from build123d import *

# Parameters (mm, degrees)
SKETCH1_W          = 432
SKETCH1_H          = 255
BASE_FLANGE1_DEPTH = 4
SKETCH4_R          = 1.75
SKETCH4_W          = 4
SKETCH4_H          = 40
SKETCH4_W_2        = 6.3
CUT_EXTRUDE1_DEPTH = 251.855037821
CUT_EXTRUDE2_DEPTH = 251.855037821
SKETCH6_R          = 1.75
CUT_EXTRUDE3_DEPTH = 251.855037821
CUT_EXTRUDE4_REACH = 252.855
SKETCH7_R          = 2.25
SKETCH8_R          = 3.25
CUT_EXTRUDE5_DEPTH = 251.855037821
CUT_EXTRUDE6_DEPTH = 251.855037821
SKETCH10_W         = 4
SKETCH10_H         = 100
CUT_EXTRUDE7_DEPTH = 251.855037821
CUT_EXTRUDE8_DEPTH = 251.855037821
SKETCH13_W         = 4
SKETCH13_H         = 20.5
TAB1_DEPTH         = 4
CUT_EXTRUDE9_REACH = 252.855


# Sheet-metal steps are written as plain solids
with BuildPart() as part:
    # Sketch1 → Base-Flange1 (new body)
    with BuildSketch(Plane.XY):
        Rectangle(SKETCH1_W, SKETCH1_H)
    extrude(amount=-BASE_FLANGE1_DEPTH)

    # Sketch4 → Cut-Extrude1 (cut, through all)
    with BuildSketch(Plane.XY):
        with Locations((-78, 82.5)):
            Circle(SKETCH4_R)
        with Locations(Location((214, -17.5, 0), (0, 0, 180))):
            Circle(SKETCH4_R)
        with Locations(Location((214, 82.5, 0), (0, 0, 180))):
            Circle(SKETCH4_R)
        with Locations((-78, -17.5)):
            Circle(SKETCH4_R)
        with Locations((-169, -17.5)):
            Circle(SKETCH4_R)
        with Locations((-169, 82.5)):
            Circle(SKETCH4_R)
        with Locations((-214, 82.5)):
            Circle(SKETCH4_R)
        with Locations((-214, -17.5)):
            Circle(SKETCH4_R)
        with Locations(Location((169, 82.5, 0), (0, 0, 180))):
            Circle(SKETCH4_R)
        with Locations(Location((169, -17.5, 0), (0, 0, 180))):
            Circle(SKETCH4_R)
        with Locations(Location((78, -17.5, 0), (0, 0, 180))):
            Circle(SKETCH4_R)
        with Locations(Location((78, 82.5, 0), (0, 0, 180))):
            Circle(SKETCH4_R)
        with Locations((-214, 32.5)):
            Rectangle(SKETCH4_W, SKETCH4_H)
        with Locations((-169, 32.5)):
            Rectangle(SKETCH4_W_2, SKETCH4_H)
        with Locations((-78, 32.5)):
            Rectangle(SKETCH4_W_2, SKETCH4_H)
        with Locations((78, 32.5)):
            Rectangle(SKETCH4_W_2, SKETCH4_H)
        with Locations((169, 32.5)):
            Rectangle(SKETCH4_W_2, SKETCH4_H)
        with Locations((214, 32.5)):
            Rectangle(SKETCH4_W, SKETCH4_H)
    extrude(amount=-CUT_EXTRUDE1_DEPTH, mode=Mode.SUBTRACT)

    # Sketch5 → Cut-Extrude2 (cut, through all)
    with BuildSketch(Plane.XY):
        with BuildLine():
            Line((-214, 80.75), (-216, 80.75))
            ThreePointArc((-216, 80.75), (-217.75, 82.5), (-216, 84.25))
            Line((-216, 84.25), (-214, 84.25))
            ThreePointArc((-214, 84.25), (-212.25, 82.5), (-214, 80.75))
        make_face()
        with BuildLine():
            Line((-214, -19.25), (-216, -19.25))
            ThreePointArc((-216, -19.25), (-217.75, -17.5), (-216, -15.75))
            Line((-216, -15.75), (-214, -15.75))
            ThreePointArc((-214, -15.75), (-212.25, -17.5), (-214, -19.25))
        make_face()
        with BuildLine():
            Line((214, 80.75), (216, 80.75))
            ThreePointArc((216, 80.75), (217.75, 82.5), (216, 84.25))
            Line((216, 84.25), (214, 84.25))
            ThreePointArc((214, 84.25), (212.25, 82.5), (214, 80.75))
        make_face()
        with BuildLine():
            Line((214, -19.25), (216, -19.25))
            ThreePointArc((216, -19.25), (217.75, -17.5), (216, -15.75))
            Line((216, -15.75), (214, -15.75))
            ThreePointArc((214, -15.75), (212.25, -17.5), (214, -19.25))
        make_face()
    extrude(amount=-CUT_EXTRUDE2_DEPTH, mode=Mode.SUBTRACT)

    # Sketch6 → Cut-Extrude3 (cut, through all)
    with BuildSketch(Plane.XY):
        with Locations((-90, -54.5)):
            Circle(SKETCH6_R)
        with Locations((90, -54.5)):
            Circle(SKETCH6_R)
    extrude(amount=-CUT_EXTRUDE3_DEPTH, mode=Mode.SUBTRACT)

    # Sketch7 → Cut-Extrude4 (cut, up to next)
    with BuildSketch(Plane.XY, mode=Mode.PRIVATE) as cut_extrude4_sk1:
        with Locations((205.5, 115.5)):
            Circle(SKETCH7_R)
    cut_extrude4_tool1 = extrude(cut_extrude4_sk1.sketch, amount=-CUT_EXTRUDE4_REACH, mode=Mode.PRIVATE) & part.part
    # Sketch7 → Cut-Extrude4 (cut, up to next)
    with BuildSketch(Plane.XY, mode=Mode.PRIVATE) as cut_extrude4_sk2:
        with Locations((205.5, 99.5)):
            Circle(SKETCH7_R)
    cut_extrude4_tool2 = extrude(cut_extrude4_sk2.sketch, amount=-CUT_EXTRUDE4_REACH, mode=Mode.PRIVATE) & part.part
    # Sketch7 → Cut-Extrude4 (cut, up to next)
    with BuildSketch(Plane.XY, mode=Mode.PRIVATE) as cut_extrude4_sk3:
        with Locations((-205.5, 99.5)):
            Circle(SKETCH7_R)
    cut_extrude4_tool3 = extrude(cut_extrude4_sk3.sketch, amount=-CUT_EXTRUDE4_REACH, mode=Mode.PRIVATE) & part.part
    # Sketch7 → Cut-Extrude4 (cut, up to next)
    with BuildSketch(Plane.XY, mode=Mode.PRIVATE) as cut_extrude4_sk4:
        with Locations((-205.5, 115.5)):
            Circle(SKETCH7_R)
    cut_extrude4_tool4 = extrude(cut_extrude4_sk4.sketch, amount=-CUT_EXTRUDE4_REACH, mode=Mode.PRIVATE) & part.part
    add(cut_extrude4_tool1.solids().sort_by_distance((205.5, 115.5, 0))[0], mode=Mode.SUBTRACT)
    add(cut_extrude4_tool2.solids().sort_by_distance((205.5, 99.5, 0))[0], mode=Mode.SUBTRACT)
    add(cut_extrude4_tool3.solids().sort_by_distance((-205.5, 99.5, 0))[0], mode=Mode.SUBTRACT)
    add(cut_extrude4_tool4.solids().sort_by_distance((-205.5, 115.5, 0))[0], mode=Mode.SUBTRACT)

    # Sketch8 → Cut-Extrude5 (cut, through all)
    with BuildSketch(Plane.XY):
        with Locations((-143.5, -67.5)):
            Circle(SKETCH8_R)
        with Locations((-103.5, -67.5)):
            Circle(SKETCH8_R)
        with Locations((-20, -67.5)):
            Circle(SKETCH8_R)
        with Locations((20, -67.5)):
            Circle(SKETCH8_R)
        with Locations((103.5, -67.5)):
            Circle(SKETCH8_R)
        with Locations((143.5, -67.5)):
            Circle(SKETCH8_R)
    extrude(amount=-CUT_EXTRUDE5_DEPTH, mode=Mode.SUBTRACT)

    # Sketch9 → Cut-Extrude6 (cut, through all)
    with BuildSketch(Plane.XY):
        with BuildLine():
            Line((-143.5, -77.5), (-103.5, -77.5))
            ThreePointArc((-103.5, -77.5), (-93.5, -87.5), (-103.5, -97.5))
            Line((-103.5, -97.5), (-143.5, -97.5))
            ThreePointArc((-143.5, -97.5), (-153.5, -87.5), (-143.5, -77.5))
        make_face()
        with BuildLine():
            Line((-20, -77.5), (20, -77.5))
            ThreePointArc((20, -77.5), (30, -87.5), (20, -97.5))
            Line((20, -97.5), (-20, -97.5))
            ThreePointArc((-20, -97.5), (-30, -87.5), (-20, -77.5))
        make_face()
        with BuildLine():
            Line((143.5, -77.5), (103.5, -77.5))
            ThreePointArc((103.5, -77.5), (93.5, -87.5), (103.5, -97.5))
            Line((103.5, -97.5), (143.5, -97.5))
            ThreePointArc((143.5, -97.5), (153.5, -87.5), (143.5, -77.5))
        make_face()
    extrude(amount=-CUT_EXTRUDE6_DEPTH, mode=Mode.SUBTRACT)

    # Sketch10 → Cut-Extrude7 (cut, through all)
    with BuildSketch(Plane.XY):
        with Locations((-214, -77.5)):
            Rectangle(SKETCH10_W, SKETCH10_H)
        with Locations((214, -77.5)):
            Rectangle(SKETCH10_W, SKETCH10_H)
    extrude(amount=-CUT_EXTRUDE7_DEPTH, mode=Mode.SUBTRACT)

    # Sketch11 → Cut-Extrude8 (cut, through all)
    with BuildSketch(Plane.XY):
        Polygon((-212, -75.75), (-209, -75.75), (-209, -74.75), (-205, -74.75), (-205, -75.75), (-200, -75.75), (-200, -79.25), (-205, -79.25), (-205, -80.25), (-209, -80.25), (-209, -79.25), (-212, -79.25), align=None)
        Polygon((212, -79.25), (212, -75.75), (209, -75.75), (209, -74.75), (205, -74.75), (205, -75.75), (200, -75.75), (200, -79.25), (205, -79.25), (205, -80.25), (209, -80.25), (209, -79.25), align=None)
    extrude(amount=-CUT_EXTRUDE8_DEPTH, mode=Mode.SUBTRACT)

    # Sketch13 → Tab1 (add)
    with BuildSketch(Plane.XY):
        with Locations((-214, -56.75)):
            Rectangle(SKETCH13_W, SKETCH13_H)
        with Locations((214, -56.75)):
            Rectangle(SKETCH13_W, SKETCH13_H)
    extrude(amount=-TAB1_DEPTH)

    # Sketch14 → Cut-Extrude9 (cut, up to next)
    with BuildSketch(Plane.XY, mode=Mode.PRIVATE) as cut_extrude9_sk1:
        with BuildLine():
            Line((-145.424403398, -70.119002016), (-141.210288019, -69.806451613))
            ThreePointArc((-141.210288019, -69.806451613), (-142.200504545, -74.714501715), (-138.039917583, -77.5))
            Line((-138.039917583, -77.5), (-146.664801345, -78.014008621))
            ThreePointArc((-146.664801345, -78.014008621), (-143.64349365, -74.443747603), (-145.424403398, -70.119002016))
        make_face()
    cut_extrude9_tool1 = extrude(cut_extrude9_sk1.sketch, amount=-CUT_EXTRUDE9_REACH, mode=Mode.PRIVATE) & part.part
    # Sketch14 → Cut-Extrude9 (cut, up to next)
    with BuildSketch(Plane.XY, mode=Mode.PRIVATE) as cut_extrude9_sk2:
        with BuildLine():
            Line((-105.789711981, -69.806451613), (-101.575596602, -70.119002016))
            ThreePointArc((-101.575596602, -70.119002016), (-103.35650635, -74.443747603), (-100.335198655, -78.014008621))
            Line((-100.335198655, -78.014008621), (-108.960082417, -77.5))
            ThreePointArc((-108.960082417, -77.5), (-104.799495455, -74.714501715), (-105.789711981, -69.806451613))
        make_face()
    cut_extrude9_tool2 = extrude(cut_extrude9_sk2.sketch, amount=-CUT_EXTRUDE9_REACH, mode=Mode.PRIVATE) & part.part
    # Sketch14 → Cut-Extrude9 (cut, up to next)
    with BuildSketch(Plane.XY, mode=Mode.PRIVATE) as cut_extrude9_sk3:
        with BuildLine():
            Line((-21.924403398, -70.119002016), (-17.710288019, -69.806451613))
            ThreePointArc((-17.710288019, -69.806451613), (-18.700504545, -74.714501715), (-14.539917583, -77.5))
            Line((-14.539917583, -77.5), (-23.164801345, -78.014008621))
            ThreePointArc((-23.164801345, -78.014008621), (-20.14349365, -74.443747603), (-21.924403398, -70.119002016))
        make_face()
    cut_extrude9_tool3 = extrude(cut_extrude9_sk3.sketch, amount=-CUT_EXTRUDE9_REACH, mode=Mode.PRIVATE) & part.part
    # Sketch14 → Cut-Extrude9 (cut, up to next)
    with BuildSketch(Plane.XY, mode=Mode.PRIVATE) as cut_extrude9_sk4:
        with BuildLine():
            Line((17.710288019, -69.806451613), (21.924403398, -70.119002016))
            ThreePointArc((21.924403398, -70.119002016), (20.14349365, -74.443747603), (23.164801345, -78.014008621))
            Line((23.164801345, -78.014008621), (14.539917583, -77.5))
            ThreePointArc((14.539917583, -77.5), (18.700504545, -74.714501715), (17.710288019, -69.806451613))
        make_face()
    cut_extrude9_tool4 = extrude(cut_extrude9_sk4.sketch, amount=-CUT_EXTRUDE9_REACH, mode=Mode.PRIVATE) & part.part
    # Sketch14 → Cut-Extrude9 (cut, up to next)
    with BuildSketch(Plane.XY, mode=Mode.PRIVATE) as cut_extrude9_sk5:
        with BuildLine():
            Line((101.575596602, -70.119002016), (105.789711981, -69.806451613))
            ThreePointArc((105.789711981, -69.806451613), (104.799495455, -74.714501715), (108.960082417, -77.5))
            Line((108.960082417, -77.5), (100.335198655, -78.014008621))
            ThreePointArc((100.335198655, -78.014008621), (103.35650635, -74.443747603), (101.575596602, -70.119002016))
        make_face()
    cut_extrude9_tool5 = extrude(cut_extrude9_sk5.sketch, amount=-CUT_EXTRUDE9_REACH, mode=Mode.PRIVATE) & part.part
    # Sketch14 → Cut-Extrude9 (cut, up to next)
    with BuildSketch(Plane.XY, mode=Mode.PRIVATE) as cut_extrude9_sk6:
        with BuildLine():
            Line((141.210288019, -69.806451613), (145.424403398, -70.119002016))
            ThreePointArc((145.424403398, -70.119002016), (143.64349365, -74.443747603), (146.664801345, -78.014008621))
            Line((146.664801345, -78.014008621), (138.039917583, -77.5))
            ThreePointArc((138.039917583, -77.5), (142.200504545, -74.714501715), (141.210288019, -69.806451613))
        make_face()
    cut_extrude9_tool6 = extrude(cut_extrude9_sk6.sketch, amount=-CUT_EXTRUDE9_REACH, mode=Mode.PRIVATE) & part.part
    add(cut_extrude9_tool1.solids().sort_by_distance((-142.940406, -74.543394, 0))[0], mode=Mode.SUBTRACT)
    add(cut_extrude9_tool2.solids().sort_by_distance((-104.059594, -74.543394, 0))[0], mode=Mode.SUBTRACT)
    add(cut_extrude9_tool3.solids().sort_by_distance((-19.440406, -74.543394, 0))[0], mode=Mode.SUBTRACT)
    add(cut_extrude9_tool4.solids().sort_by_distance((19.440406, -74.543394, 0))[0], mode=Mode.SUBTRACT)
    add(cut_extrude9_tool5.solids().sort_by_distance((104.059594, -74.543394, 0))[0], mode=Mode.SUBTRACT)
    add(cut_extrude9_tool6.solids().sort_by_distance((142.940406, -74.543394, 0))[0], mode=Mode.SUBTRACT)


solid = part.part
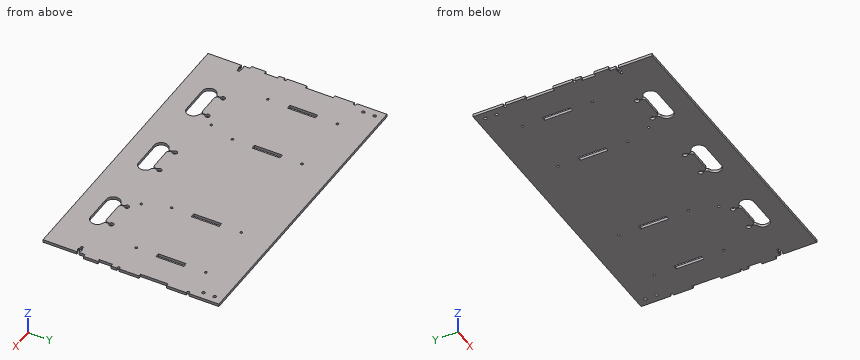
The model under review builds one solid part; all positions refer to its coordinate system, in mm. Give positions to 0.01 mm unless a question says otherwise; leave off trailing zeros. Order: outer loops, then holes, each group sorted by start corner. A loop starts at its lowest first (then second) coordinate and runs counter-clockwise, first axis right, second up. Notation, with made-up numbers: M -2.75,-16 L 46.25,-16 A20 ccw 46.25,-8 Z; hole C 31,26 d2. An arc over 180 degrees is marked long. Use one line per item in the form item = value. Start each with the question number.
Item 1: We need section A-A on y = -36. Give the boundary of the cut face in (x, z).
Item 2: Insertion check: pin 1 Ø1.1 at (y, z) = (-75, -2) entering from -X. The pin has a flat end and moves straight along its axis. Give the tip position at first contact, or say it passes through.
Item 3: To check wall thickness, follow line 1 along Y through (x, z) = (78, -2.45); line 2 along X through (y, z) = (82.5, -1.45); line 3 along Y through (x, z) = (-20, -3.15). State the ranges of each line that lie inside material, in increasing order. Write a range as from..to.
Item 4: We need section B-B on z = -1.25. Give the number of separate pieces and of enclosed holes in the cut face, plus the area to 3 significant figures.
Completed:
q1.outline = M -212,-4 L 212,-4 L 212,0 L -212,0 Z
q2.pin_1 = -212
q3.line_1 = -127.5..-19.25, -15.75..12.5, 52.5..80.75, 84.25..127.5
q3.line_2 = -212.25..-170.75, -167.25..-79.75, -76.25..76.25, 79.75..167.25, 170.75..212.25
q3.line_3 = -127.5..-97.5, -64.25..127.5
q4.separate_pieces = 1
q4.enclosed_holes = 21
q4.area = 104,000 mm²
